Read the model definition and answer for the solid it produces. Units are mm, in the model's axes. Give positions to 0.01 mm unless a question says otherwise; leave off trailing zeros. Order: outer loops, then holes, each group sorted by start corner. A loop starts at its lowest first (then second) coordinate and runs counter-clockwise, first axis right, second up.
Item 1: Find the intervals of material crossed by line 1 along Y through (x, z) = (0, 3.8); line 2 along X through (y, z) = (5.5, 2.8), in increasing order.
Item 2: Given pin 1 Ø0.6 at (x, z) = (-15, 2.5) entering from +Y; pin 2 Ø1.5 at (x, z) = (-7, 3.5) entering from -Y; pin 3 Ø0.6 at (y, z) = (5.5, 2.5) entering from +X, each flat-ended and moving along its own axis, determine where each tip first touches the part or whether it passes through.
Item 3: A cutting plane is placed at C-C (z = 2.65). Write down the section's boundary in (x, y).
Item 4: A cutting plane is placed at A-A (y = -15). Write down the section's boundary in (x, z), plus the area to 3 significant figures.
Item 5: A cutting plane is placed at B-B (x = 10.5). Write down the section's boundary in (y, z), plus the area to 3 significant figures.
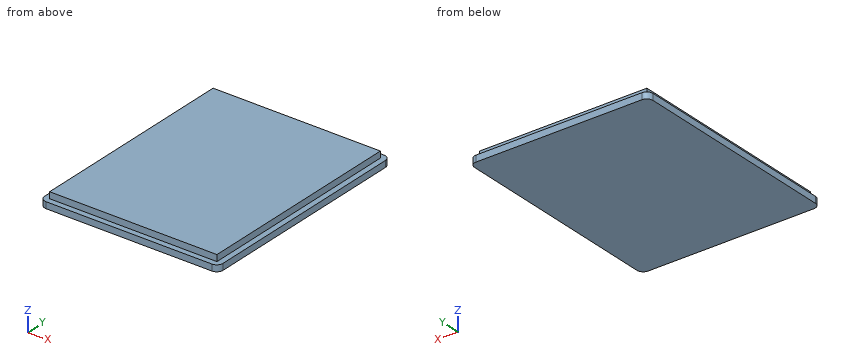
from build123d import *

# Parameters (mm, degrees)
F0_W     = 56.021
F0_H     = 70.122
F0_W_2   = 52.521
F0_H_2   = 66.622
F1_DEPTH = 2
F2_R     = 2
F3_DEPTH = 4


with BuildPart() as f1:
    # F0 (on Top) → F1 (new body)
    with BuildSketch(Plane.XY):
        with Locations((-9.772905, 4.139024)):
            Rectangle(F0_W, F0_H)
        with Locations((-9.772905, 4.139024)):
            Rectangle(F0_W_2, F0_H_2, mode=Mode.SUBTRACT)
    extrude(amount=F1_DEPTH)

    # F2
    f2_edges = [f1.edges().sort_by_distance(p)[0] for p in [
        (-37.783405, -30.921976, 1),
        (-37.783405, 39.200024, 1),
        (18.237595, 39.200024, 1),
        (18.237595, -30.921976, 1),
    ]]
    fillet(f2_edges, radius=F2_R)

    # F0 (on Top) → F3 (join)
    with BuildSketch(Plane.XY):
        with Locations((-9.772905, 4.139024)):
            Rectangle(F0_W_2, F0_H_2)
    extrude(amount=F3_DEPTH)


solid = f1.part
Response values:
1. line 1: y = -29.17 to 37.45
1. line 2: x = -36.03 to 16.49
2. pin 1: stops at y = 37.45
2. pin 2: stops at y = -29.17
2. pin 3: stops at x = 16.49
3. outline: (-36.03, -29.17) - (16.49, -29.17) - (16.49, 37.45) - (-36.03, 37.45) - close
4. outline: (-37.78, 0) - (18.24, 0) - (18.24, 2) - (16.49, 2) - (16.49, 4) - (-36.03, 4) - (-36.03, 2) - (-37.78, 2) - close
4. area: 217 mm2
5. outline: (-30.92, 0) - (39.2, 0) - (39.2, 2) - (37.45, 2) - (37.45, 4) - (-29.17, 4) - (-29.17, 2) - (-30.92, 2) - close
5. area: 273 mm2
